For this review, take the finished solid that the model builds, in its own axes (mm). Face numbers are marked on the shaded views. A direction names the side the tool comes from. Coordinates: 2 decimals unless noted, no trailing zeros. Order: outer loops, then holes, each group sorted by start corner. A loop starts at its lowest first (then second) coordinate and runs counter-clockwise, first axis right, second up. Notation, with made-up numbers: M 32,52.5 L 38,52.5 A14 ccw 38,58.5 Z; hole C -33.5,-38 d7. An arc over 180 degrees is marked long. Use CSV: the item, a comma, the result in double quotes.
```python
from build123d import *

# Parameters (mm, degrees)
ESQUISSE1_W                  = 45
ESQUISSE1_H                  = 35
BOSS_EXTRU_1_DEPTH           = 6
ESQUISSE2_R                  = 3
ENL_V_MAT_EXTRU_1_DEPTH      = 7
ESQUISSE3_W                  = 8.2
ESQUISSE3_H                  = 16.2
ENL_V_MAT_EXTRU_2_DEPTH      = 7
ESQUISSE4_W                  = 35
ESQUISSE4_H                  = 10
BOSS_EXTRU_2_DEPTH           = 6.5
ESQUISSE5_W                  = 35
ESQUISSE5_H                  = 10
BOSS_EXTRU_3_DEPTH           = 6.5
ESQUISSE7_W                  = 11
ESQUISSE7_H                  = 10
BOSS_EXTRU_4_DEPTH           = 9
ESQUISSE8_W                  = 11
ESQUISSE8_H                  = 10
BOSS_EXTRU_5_DEPTH           = 9
ESQUISSE6_R                  = 1.6
ENL_V_MAT_EXTRU_3_DEPTH      = 12.9
ENL_V_MAT_EXTRU_3_DEPTH_BACK = 34.1


with BuildPart() as part:
    # Esquisse1 → Boss.-Extru.1 (new body)
    with BuildSketch(Plane(origin=(0, 0, 0), x_dir=(1, 0, 0), z_dir=(0, 1, 0))):
        with Locations((0, 1)):
            Rectangle(ESQUISSE1_W, ESQUISSE1_H)
    extrude(amount=BOSS_EXTRU_1_DEPTH)

    # Esquisse2 → Enlèv. mat.-Extru.1 (cut, through all)
    with BuildSketch(Plane(origin=(0, 6, 0), x_dir=(1, 0, 0), z_dir=(0, 1, 0))):
        with Locations((-15.5, 13.5)):
            Circle(ESQUISSE2_R)
        with Locations((-15.5, -11.5)):
            Circle(ESQUISSE2_R)
        with Locations((15.5, -11.5)):
            Circle(ESQUISSE2_R)
        with Locations((15.5, 13.5)):
            Circle(ESQUISSE2_R)
    extrude(amount=-ENL_V_MAT_EXTRU_1_DEPTH, mode=Mode.SUBTRACT)

    # Esquisse3 → Enlèv. mat.-Extru.2 (cut, through all)
    with BuildSketch(Plane(origin=(0, 6, 0), x_dir=(1, 0, 0), z_dir=(0, 1, 0))):
        Rectangle(ESQUISSE3_W, ESQUISSE3_H)
    extrude(amount=-ENL_V_MAT_EXTRU_2_DEPTH, mode=Mode.SUBTRACT)

    # Esquisse4 → Boss.-Extru.2 (add)
    with BuildSketch(Plane(origin=(-4.1, 0, 0), x_dir=(0, 0, -1), z_dir=(1, 0, 0))):
        with Locations((1, 11)):
            Rectangle(ESQUISSE4_W, ESQUISSE4_H)
    extrude(amount=-BOSS_EXTRU_2_DEPTH)

    # Esquisse5 → Boss.-Extru.3 (add)
    with BuildSketch(Plane(origin=(4.1, 0, -4), x_dir=(0, 0, 1), z_dir=(-1, 0, 0))):
        with Locations((3, 11)):
            Rectangle(ESQUISSE5_W, ESQUISSE5_H)
    extrude(amount=-BOSS_EXTRU_3_DEPTH)

    # Esquisse7 → Boss.-Extru.4 (add)
    with BuildSketch(Plane(origin=(10.6, 0, 0), x_dir=(0, 0, -1), z_dir=(1, 0, 0))):
        with Locations((1, 11)):
            Rectangle(ESQUISSE7_W, ESQUISSE7_H)
    extrude(amount=BOSS_EXTRU_4_DEPTH)

    # Esquisse8 → Boss.-Extru.5 (add)
    with BuildSketch(Plane(origin=(-10.6, 0, -10.5), x_dir=(0, 0, -1), z_dir=(1, 0, 0))):
        with Locations((-9.5, 11)):
            Rectangle(ESQUISSE8_W, ESQUISSE8_H)
    extrude(amount=-BOSS_EXTRU_5_DEPTH)

    # Esquisse6 → Enlèv. mat.-Extru.3 (cut, two sides)
    with BuildSketch(Plane(origin=(10.6, 0, 0), x_dir=(0, 0, -1), z_dir=(1, 0, 0))) as enl_v_mat_extru_3_sk:
        with Locations((0, 9.2)):
            Circle(ESQUISSE6_R)
    extrude(amount=ENL_V_MAT_EXTRU_3_DEPTH, mode=Mode.SUBTRACT)
    extrude(enl_v_mat_extru_3_sk.sketch, amount=-ENL_V_MAT_EXTRU_3_DEPTH_BACK, mode=Mode.SUBTRACT)


solid = part.part
```
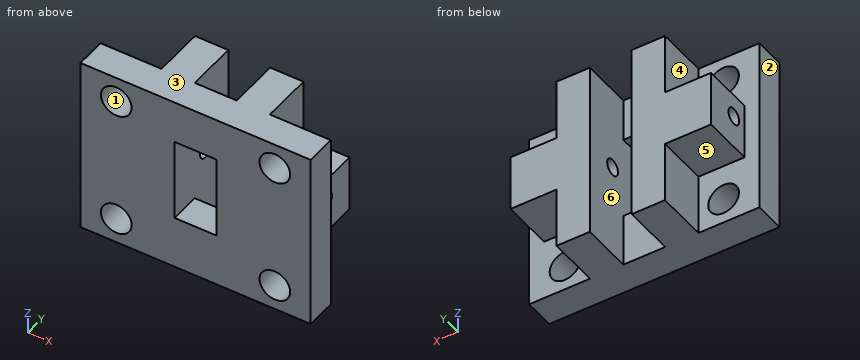
Item 1: Add section A-A on x = 15.5. State the section outline as (y, z) points, and give its area (3 significant figures).
Solutions:
outline,"M 0,-18.5 L 6,-18.5 L 6,-16.5 L 0,-16.5 Z; M 0,-10.5 L 6,-10.5 L 6,-6.5 L 16,-6.5 L 16,4.5 L 6,4.5 L 6,8.5 L 0,8.5 Z; M 0,14.5 L 6,14.5 L 6,16.5 L 0,16.5 Z; hole C 9.2,0 d3.2"
area,"240 mm^2"
Item 2: Clearance check with flat-ended pins moving along their axes: pin 1 Ø5 at (y, z) = (11.5, 0.5) entering from -X; pin 2 Ø4 at (x, z) = (2, -11) entering from +Y; pin 3 Ø8 at (x, y) = (16, 14) entering from +Z. State where each tip first meets the part, or that it passes through.
Solutions:
pin 1,"x = -19.6"
pin 2,"y = 6"
pin 3,"z = 4.5"
Item 3: To check wall thickness, follow line 1 along Z through (x, y) = (-15.5, 3.4); line 2 along X through (y, z) = (2.25, -13.5); line 3 along X through (y, z) = (11, 5.5). State the ranges of each line that lie inside material, in increasing order. Write a range as [from, to].
Solutions:
line 1,"[-18.5, -16.5], [-10.5, 8.5], [14.5, 16.5]"
line 2,"[-22.5, -18.5], [-12.5, 12.5], [18.5, 22.5]"
line 3,"[-10.6, -4.1], [4.1, 10.6]"
Item 4: Add section B-B on z = 0. State the section outline as (x, y) points, and give its area (3 significant figures).
Solutions:
outline,"M -22.5,0 L -4.1,0 L -4.1,7.6 L -19.6,7.6 L -19.6,6 L -22.5,6 Z; M -19.6,10.8 L -4.1,10.8 L -4.1,16 L -19.6,16 Z; M 4.1,0 L 22.5,0 L 22.5,6 L 19.6,6 L 19.6,7.6 L 4.1,7.6 Z; M 4.1,10.8 L 19.6,10.8 L 19.6,16 L 4.1,16 Z"
area,"432 mm^2"
Item 5: For the marked faces 4, 5 and 6, list the 3-axis set-ups (+Z, -Z, +X, -X, +Y, -Y) from which the entire face can be reached by the end or side of a thin tool; tool diameter is ignored.
Solutions:
face 4,"+Z, -X, +Y"
face 5,"-Z, -X, +Y"
face 6,"+Y"
Item 6: Add section D-D on y = 14.75. State the section outline as (x, z) points, and give its area (3 significant figures).
Solutions:
outline,"M -19.6,-6.5 L -10.6,-6.5 L -10.6,-18.5 L -4.1,-18.5 L -4.1,16.5 L -10.6,16.5 L -10.6,4.5 L -19.6,4.5 Z; M 4.1,-18.5 L 10.6,-18.5 L 10.6,-6.5 L 19.6,-6.5 L 19.6,4.5 L 10.6,4.5 L 10.6,16.5 L 4.1,16.5 Z"
area,"653 mm^2"
Item 7: Add section C-C on z = 7. State the section outline as (x, y) points.
Solutions:
outline,"M -22.5,0 L -4.1,0 L -4.1,16 L -10.6,16 L -10.6,6 L -22.5,6 Z; M 4.1,0 L 22.5,0 L 22.5,6 L 10.6,6 L 10.6,16 L 4.1,16 Z"
Item 8: Draft analysis for pull direction X (two halves, no side actions). For the marked faces 1, 2 and 3, state which applies: released by +X, released by -X, zero draft, split by the parting line, or undercut.
Solutions:
face 1,"undercut"
face 2,"released by -X"
face 3,"zero draft"
